The drawing under review shows one solid part. Ordinate dimensions are in mm from its lowest x, y, z. Coordinates: 2 decimals unless noted, no trailing zeros. Write each loop counter-clockwise with the first axis right and the second up, starting at its lowest first coordinate (ties: lowest second). Pieces come first, ordered by that corner, then holes. Notation, with made-up numbers: (61.25, 30) - (102.25, 30) arc R16 ccw to (102.25, 57) - close; hole circle Ø11 at (22, 32). An arc over 180 degrees is marked (long way). Answer as CSV lines item,"result". Start each with the question number.
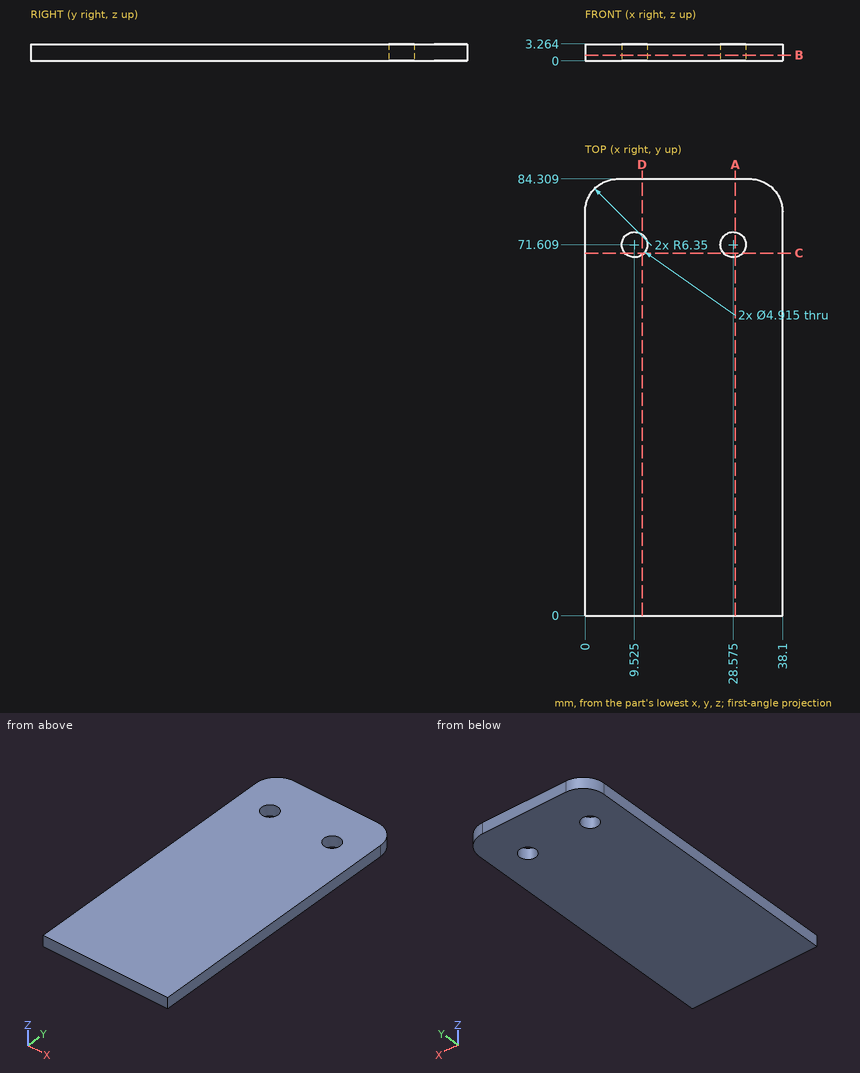
(1) Wall thickness on line 1 (X direction, y = 81, z = 2.3); line 2 (Y direction, x = 3, z = 2.4); line 3 (Y direction, x = 4, z = 1.2): over which ranges is each line inside the solid? List them lowest first.
(2) Add section C-C on y = 70. Give the boundary of the cut face in (x, z), then the cut area to 3 significant figures.
(3) Add section B-B on z = 1.1. Give the number of separate pieces and of enclosed holes in the cut face, then the cut area to 3 significant figures.
(4) Add section D-D on x = 11. Give the boundary of the cut face in (y, z), then the cut area to 3 significant figures.
(5) Add section A-A on x = 29. Give the boundary of the cut face in (y, z), then the cut area to 3 significant figures.
Reported:
1,line 1,"0.78 to 37.32"
1,line 2,"0 to 83.35"
1,line 3,"0 to 83.86"
2,outline,"(0, 0) - (7.67, 0) - (7.67, 3.26) - (0, 3.26) - close; (11.38, 0) - (26.72, 0) - (26.72, 3.26) - (11.38, 3.26) - close; (30.43, 0) - (38.1, 0) - (38.1, 3.26) - (30.43, 3.26) - close"
2,area,"100 mm²"
3,separate pieces,"1"
3,enclosed holes,"2"
3,area,"3,160 mm²"
4,outline,"(0, 0) - (69.64, 0) - (69.64, 3.26) - (0, 3.26) - close; (73.57, 0) - (84.31, 0) - (84.31, 3.26) - (73.57, 3.26) - close"
4,area,"262 mm²"
5,outline,"(0, 0) - (69.19, 0) - (69.19, 3.26) - (0, 3.26) - close; (74.03, 0) - (84.31, 0) - (84.31, 3.26) - (74.03, 3.26) - close"
5,area,"259 mm²"
